Autodesk Inventor part; units mm, degrees
ref_plane "YZ Plane" through (0, 0, 0) normal (1, 0, 0) x (0, 1, 0)
ref_plane "XZ Plane" through (0, 0, 0) normal (0, 1, 0) x (-1, 0, 0)
ref_plane "XY Plane" through (0, 0, 0) normal (0, 0, 1) x (1, 0, 0)
ref_plane "Work Plane1" through (92.6217, 101.5189, 36.552) normal (1, 0, 0) x (0, 1, 0)
ref_plane "Work Plane2" through (89.5017, 946.6624, 79.752) normal (0, 0, 1) x (0.6133, 0.7899, 0)
sketch "Sketch1" plane through (92.6217, 101.5189, 36.552) normal (1, 0, 0) x (0, 1, 0)
  line L0 (31.35, 24.7) -> (31.35, 16.2)
  line L1 (31.35, 16.2) -> (9.35, 16.2)
  line L2 (9.35, 16.2) -> (9.35, 24.7)
  line L3 (0, 24.7) -> (9.35, 24.7)
  line L4 (0, 0) -> (0, 24.7) construction
  line L5 (40.7, 0) -> (0, 0)
  line L6 (40.7, 0) -> (40.7, 24.7)
  line L7 (31.35, 24.7) -> (40.7, 24.7)
  line L8 (9.35, 61.7) -> (9.35, 70.2)
  line L9 (9.35, 70.2) -> (31.35, 70.2)
  line L10 (31.35, 70.2) -> (31.35, 61.7)
  line L11 (31.35, 61.7) -> (40.7, 61.7)
  line L12 (40.7, 61.7) -> (40.7, 86.4)
  line L13 (40.7, 86.4) -> (0, 86.4)
  line L14 (0, 86.4) -> (0, 61.7) construction
  line L15 (0, 61.7) -> (9.35, 61.7)
  line L16 (-4.1716, 58.2) -> (44.8716, 58.2)
  line L17 (-4.1716, 28.2) -> (44.8716, 28.2)
  line L18 (-300, 136.4) -> (-300, 120.8667)
  line L19 (0, 61.7) -> (-4.1716, 61.7)
  line L20 (-4.1716, 61.7) -> (-7.6716, 61.7)
  line L21 (-7.6716, 61.7) -> (-7.6716, 43.2)
  line L22 (-4.1716, 58.2) -> (-4.1716, 61.7) construction
  line L23 (-372.5743, 43.2) -> (114.4459, 43.2) construction
  line L24 (0, 24.7) -> (-4.1716, 24.7)
  line L25 (-4.1716, 24.7) -> (-7.6716, 24.7)
  line L26 (-7.6716, 24.7) -> (-7.6716, 43.2)
  line L27 (0, 86.4) -> (-3, 86.4)
  line L28 (-3, 86.4) -> (-3, 96.4)
  line L29 (-3, 96.4) -> (-300, 136.4)
  line L30 (0, 0) -> (-3, 0)
  line L31 (-3, 0) -> (-3, -10)
  line L32 (-300, 120.8667) -> (-303, 120.8667)
  line L33 (-303, 120.8667) -> (-303, 89.8)
  line L34 (-303, 89.8) -> (-300, 89.8)
  line L35 (-300, 89.8) -> (-300, 58.7333)
  line L36 (-300, 58.7333) -> (-303, 58.7333)
  line L37 (-303, 58.7333) -> (-303, 27.6667)
  line L38 (-303, 27.6667) -> (-300, 27.6667)
  line L39 (-300, 27.6667) -> (-300, -3.4)
  line L40 (-300, -3.4) -> (-303, -3.4)
  line L41 (-303, -3.4) -> (-303, -34.4667)
  line L42 (-303, -34.4667) -> (-300, -34.4667)
  line L43 (-300, -34.4667) -> (-300, -50)
  line L44 (-300, -50) -> (-3, -10)
  point P0 (-101.5189, -36.552)
  dimension "d2" = 10
  dimension "d4" = 3
extrude "Extrusion1" add sketch "Sketch1" along normal blind 3
sketch "Sketch2" plane through (95.6217, 101.5189, 36.552) normal (1, 0, 0) x (0, 0, -1)
  line L0 (-24.7, 40.7) -> (-24.7, 31.35)
  line L1 (-24.7, 31.35) -> (-16.2, 31.35)
  line L2 (-16.2, 31.35) -> (-16.2, 9.35)
  line L3 (-16.2, 9.35) -> (-24.7, 9.35)
  line L4 (-24.7, 9.35) -> (-24.7, -7.6716)
  line L5 (-24.7, -7.6716) -> (-61.7, -7.6716)
  line L6 (-61.7, -7.6716) -> (-61.7, 9.35)
  line L7 (-61.7, 9.35) -> (-70.2, 9.35)
  line L8 (-70.2, 9.35) -> (-70.2, 31.35)
  line L9 (-70.2, 31.35) -> (-61.7, 31.35)
  line L10 (-61.7, 31.35) -> (-61.7, 40.7)
  line L11 (-61.7, 40.7) -> (-86.4, 40.7)
  line L12 (-86.4, 40.7) -> (-86.4, -3)
  line L13 (-86.4, -3) -> (-96.4, -3)
  line L14 (-96.4, -3) -> (-136.4, -300)
  line L15 (-136.4, -300) -> (-120.8667, -300)
  line L16 (-120.8667, -300) -> (-120.8667, -303)
  line L17 (-120.8667, -303) -> (-89.8, -303)
  line L18 (-89.8, -303) -> (-89.8, -300)
  line L19 (-89.8, -300) -> (-58.7333, -300)
  line L20 (-58.7333, -300) -> (-58.7333, -303)
  line L21 (-58.7333, -303) -> (-27.6667, -303)
  line L22 (-27.6667, -303) -> (-27.6667, -300)
  line L23 (-27.6667, -300) -> (3.4, -300)
  line L24 (3.4, -300) -> (3.4, -303)
  line L25 (3.4, -303) -> (34.4667, -303)
  line L26 (34.4667, -303) -> (34.4667, -300)
  line L27 (34.4667, -300) -> (50, -300)
  line L28 (50, -300) -> (10, -3)
  line L29 (10, -3) -> (0, -3)
  line L30 (0, -3) -> (0, 40.7)
  line L31 (0, 40.7) -> (-24.7, 40.7)
  point P0 (36.552, -101.5189)
properties part number "Stand 2" material "Wood (Oak)"
Can you work these out from the model? Positions are in its coordinate system, mm. Round coordinates to 2 decimals unless told otherwise and drop trailing zeros. Write each loop counter-clockwise with the first axis right and the second up, starting at its lowest first coordinate (ties: lowest second). Pieces come first, ordered by that corner, then holes. Notation, with made-up numbers: M -34.75,15 L -25.75,15 A25 cw -25.75,50 Z; hole C 70.25,8.25 d5. An arc over 180 degrees is marked long. Use CSV: the item, a comma, the result in double quotes.
(1) Imagine slicing it at C-C (z = 78). Write out the boundary of the cut face in (x, y), plus the area to 3 significant figures.
Check values:
outline,"M 92.62,-201.48 L 95.62,-201.48 L 95.62,93.85 L 92.62,93.85 Z"
area,"886 mm^2"
(2) Imagine slicing it at A-A (y = 106.5). Write out the boundary of the cut face in (x, z).
Check values:
outline,"M 92.62,36.55 L 95.62,36.55 L 95.62,61.25 L 92.62,61.25 Z; M 92.62,98.25 L 95.62,98.25 L 95.62,122.95 L 92.62,122.95 Z"
(3) I need wall thicknesses on line 1 along Z through (x, y) = (93.05, 125); line 2 along Y through (x, z) = (94.4, 55); line 3 along Y through (x, z) = (94.15, 76). Which ranges of each line are inside material? Lowest first, please.
Check values:
line 1,"36.55 to 52.75, 106.75 to 122.95"
line 2,"-198.48 to 110.87, 132.87 to 142.22"
line 3,"-201.48 to 93.85"
(4) I'm going to push flat-ended pins straight in: pin 1 (0.9 mm diameter, centred on x = 93.5, y = -200.5, fed in from +Z); pin 2 (0.9 mm diameter, centred on x = 94, y = 122.5, fed in from +Z); pin 3 (0.9 mm diameter, centred on x = 94, y = 112.5, fed in from -Z). Where does each tip first touch, or does it pass through?
Check values:
pin 1,"z = 157.42"
pin 2,"z = 122.95"
pin 3,"z = 36.55"
(5) Imagine slicing it at D-D (y = -18.5). Write out the boundary of the cut face in (x, z).
Check values:
outline,"M 92.62,10.79 L 95.62,10.79 L 95.62,148.71 L 92.62,148.71 Z"
